Here's how the part is built. I have some questions about the finished solid (model axes, mm). Face numbers are marked on the shaded views. A direction names the side the tool comes from. Round coordinates to 2 decimals unless told otherwise and drop trailing zeros. Loops run counter-clockwise (first coordinate to the right, second up) from the corner with the lowest first, then second, coordinate; pieces in that order, holes last. Notation, with made-up numbers: (-11, 36) -> (24, 36) arc R27 cw to (24, 57) -> close; hole circle Ø11 at (43.25, -16). An arc over 180 degrees is marked (long way). Use CSV: the item, a comma, the result in double quotes. Start each with the question number.
from build123d import *

# Parameters (mm, degrees)
EXTRUDE_1_DEPTH = 10
EXTRUDE_START   = 47
SKETCH_6_R      = 2
EXTRUDE_2_DEPTH = 8
EXTRUDE_START_2 = -39
SKETCH_6_2_R    = 2
EXTRUDE_3_DEPTH = 8
CHAMFER_2_SIZE  = 2
SKETCH_7_R      = 2
EXTRUDE_4_DEPTH = 5
CHAMFER_3_SIZE  = 3


with BuildPart() as part:
    # 草图1 → 凸台-拉伸1 (new body)
    with BuildSketch(Plane(origin=(0, 0, 0), x_dir=(1, 0, 0), z_dir=(0, 1, 0))):
        Polygon((-47, 0), (47, 0), (47, -8), (4, -8), (4, -12), (10, -12), (10, -20), (-10, -20), (-10, -12), (-4, -12), (-4, -8), (-47, -8), align=None)
    extrude(amount=EXTRUDE_1_DEPTH)

    # 草图6 → 凸台-拉伸2 (add)
    with BuildSketch(Plane(origin=(0, 0, 0), x_dir=(0, 0, -1), z_dir=(1, 0, 0)).offset(EXTRUDE_START)):
        with BuildLine():
            Line((0.868240888, 9.924038765), (15.640357184, 7.3193161))
            ThreePointArc((15.640357184, 7.3193161), (19.69615506, 1.527036447), (13.903875407, -2.52876143))
            Line((13.903875407, -2.52876143), (-0.868240888, 0.075961235))
            ThreePointArc((-0.868240888, 0.075961235), (-4.924038765, 5.868240888), (0.868240888, 9.924038765))
        make_face()
        with Locations(Location((14.772116295, 2.395277335, 0), (0, 0, 180))):
            Circle(SKETCH_6_R, mode=Mode.SUBTRACT)
    extrude(amount=-EXTRUDE_2_DEPTH)

    # 草图6<2> → 凸台-拉伸3 (add)
    with BuildSketch(Plane(origin=(0, 0, 0), x_dir=(0, 0, -1), z_dir=(1, 0, 0)).offset(EXTRUDE_START_2)):
        with BuildLine():
            Line((0.868240888, 9.924038765), (15.640357184, 7.3193161))
            ThreePointArc((15.640357184, 7.3193161), (19.69615506, 1.527036447), (13.903875407, -2.52876143))
            Line((13.903875407, -2.52876143), (-0.868240888, 0.075961235))
            ThreePointArc((-0.868240888, 0.075961235), (-4.924038765, 5.868240888), (0.868240888, 9.924038765))
        make_face()
        with Locations(Location((14.772116295, 2.395277335, 0), (0, 0, 180))):
            Circle(SKETCH_6_2_R, mode=Mode.SUBTRACT)
    extrude(amount=-EXTRUDE_3_DEPTH)

    # 倒角2
    chamfer_2_edges = [part.edges().sort_by_distance(p)[0] for p in [
        (10, 5, 12),
        (-10, 5, 12),
    ]]
    chamfer(chamfer_2_edges, length=CHAMFER_2_SIZE)

    # 草图7 → 凸台-拉伸4 (add)
    with BuildSketch(Plane.ZY.offset(10)):
        with BuildLine():
            Line((20, 10), (44, 10))
            ThreePointArc((44, 10), (49, 5), (44, 0))
            Line((44, 0), (20, 0))
            ThreePointArc((20, 0), (15, 5), (20, 10))
        make_face()
        with Locations((44, 5)):
            Circle(SKETCH_7_R, mode=Mode.SUBTRACT)
    extrude_4 = extrude(amount=-EXTRUDE_4_DEPTH)

    # 镜向1: 凸台-拉伸4 across plane
    add(extrude_4.mirror(Plane(origin=(0, 0, 0), x_dir=(0, 0, 1), z_dir=(1, 0, 0))))

    # 倒角3
    chamfer_3_edges = [part.edges().sort_by_distance(p)[0] for p in [
        (0, 0, 20),
        (0, 10, 20),
    ]]
    chamfer(chamfer_3_edges, length=CHAMFER_3_SIZE)


solid = part.part
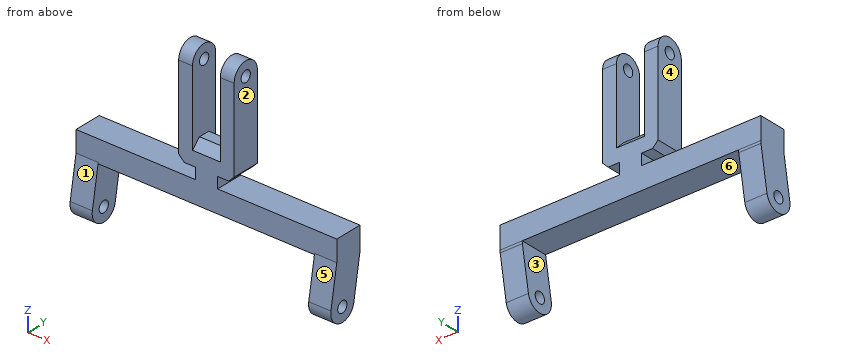
Q1. I want a section at C-C, the plane x = 41.5. List the corners of the cut face in (y, z) for me.
Q2. I want a section at D-D, the plane z = 5.5. List the corners of the cut face in (x, y) for me.
Q3. I need wall thicknesses on line 1 along Y through (x, z) = (-6.1, 44); line 2 along X through (y, z) = (9, 30); line 3 along Z through (x, y) = (-38.5, 2.5). Which ranges of each line are inside material? Lowest first, please.
Q4. I want a section at B-B, the plane z = 39. List the corners of the cut face in (x, y) for me.
Q5. If we mould it in two halves opening along X, with no side actions, what happens to the marked faces 4, 5 and 6? For each: pulls with the +X half, pulls with the -X half, needs draft (parallel to the pull), parting line crosses it, or undercut.
Q6. I want a section at A-A, the plane x = -6. List the corners of the cut face in (y, z) for me.
Q7. Will these pins go through, and if not, where does the flat tip stop? pin 1 Ø1.2 at (y, z) = (2.5, 10.5) entering from -X; pin 2 Ø6 at (y, z) = (2, 36.5) entering from -X; pin 3 Ø6 at (x, y) = (36.5, 5.5) entering from +Z.
Q8. For the marked faces 1, 2 and 3, which set-ups out of +Z, -Z, +X, -X, +Y, -Y let a thin tool reach every point of the face, with its end or its side?
Values found:
1,outline,"(-2.53, -13.9) arc R5 ccw to (7.32, -15.64) -> (9.92, -0.87) arc R5 ccw to (10, 0) -> (10, 8) -> (0, 8) -> (0, 0.44) -> close; hole circle Ø4 at (2.4, -14.77)"
2,outline,"(-47, 0) -> (47, 0) -> (47, 10) -> (-47, 10) -> close"
3,line 1,"0 to 3, 7 to 10"
3,line 2,"-10 to -5, 5 to 10"
3,line 3,"0 to 8"
4,outline,"(-10, 0) -> (-5, 0) -> (-5, 10) -> (-10, 10) -> close; (5, 0) -> (10, 0) -> (10, 10) -> (5, 10) -> close"
5,face 4,"pulls with the -X half"
5,face 5,"needs draft"
5,face 6,"undercut"
6,outline,"(0, 0) -> (10, 0) -> (10, 8) -> (0, 8) -> close; (0, 12) -> (10, 12) -> (10, 44) arc R5 ccw to (0, 44) -> close; hole circle Ø4 at (5, 44)"
7,pin 1,"x = -4"
7,pin 2,"x = -10"
7,pin 3,"z = 8"
8,face 1,"+Z, +X, -X, -Y"
8,face 2,"+Z, +X, +Y, -Y"
8,face 3,"-Z, +Y, -Y"
